from build123d import *

# Parameters (mm, degrees)
F0_W     = 75
F0_H     = 75
F1_DEPTH = 1125
F2_SIZE2 = 20.096179
F2_SIZE  = 74.99999


# Not quite as in the source:
# - a fillet or chamfer is up to 0.001 mm smaller than in the source, because OpenCascade refuses the exact size


with BuildPart() as f1:
    # F0 (on Front) → F1 (new body)
    with BuildSketch(Plane.XZ):
        Rectangle(F0_W, F0_H)
    extrude(amount=F1_DEPTH)

    # F2 (size 75 and 20.0961894323 in the source; OpenCascade refuses exactly that, so slightly less here)
    f2_edges = [f1.edges().sort_by_distance(p)[0] for p in [
        (37.5, -1125, 0),
        (0, -1125, -37.5),
    ]]
    f2_side = f1.faces().sort_by_distance((0, -1125, 0))[0]
    chamfer(f2_edges, length=F2_SIZE, length2=F2_SIZE2, reference=f2_side)


solid = f1.part
Here's how the part is built. I have some questions about the finished solid (model axes, mm). Coordinates: 2 decimals unless noted, no trailing zeros. Order: outer loops, then holes, each group sorted by start corner. A loop starts at its lowest first (then second) coordinate and runs counter-clockwise, first axis right, second up. Notation, with made-up numbers: M -33.75,34 L -20.75,34 A29 cw -20.75,55 Z; hole C -0.75,33.5 d2. An arc over 180 degrees is marked long. Answer as CSV lines item,"result".
Item 1: For pin 1 (1 mm diameter, centred on x = 20.5, z = 2, fed in from -Y); pin 2 (2 mm diameter, centred on x = 29.5, z = -27.5, fed in from -Y), each with a flat end and sliding along its axis, tell me the tip position at first contact or that it passes through.
Results found:
pin 1,"y = -1109.59"
pin 2,"y = -1107.32"
Item 2: Imagine slicing it at A-A on z = -27. Write out the boundary of the cut face in (x, y), plus the area to 3 significant figures.
Results found:
outline,"M -37.5,-1107.72 L 27,-1107.72 L 37.5,-1104.9 L 37.5,0 L -37.5,0 Z"
area,"83,100 mm2"
Item 3: If I drill on line 1 (Y direction, x = 18.5, z = -34); line 2 (Y direction, x = 25.5, z = -11), over which ranges is the centre line in solid material (lowest first)?
Results found:
line 1,"-1105.84 to 0"
line 2,"-1108.12 to 0"
